Can you work these out from the model? Positions are in its coordinate system, mm. Face numbers are marked on the shaded views. Round coordinates to 2 decimals unless told otherwise and drop trailing zeros. Write each loop counter-clockwise with the first axis right and the second up, starting at its lowest first coordinate (ties: lowest second). Pieces come first, ordered by that corner, then holes.
Q1. I'm going to push flat-ended pins straight in: pin 1 Ø1.5 at (x, z) = (6.5, -12) entering from +Y; pin 2 Ø5 at (x, z) = (-2, -4) entering from +Y; pin 3 Ø5 at (y, z) = (7.5, -4.5) entering from -X. Where does each tip first touch, or does it pass through?
Q2. If we section it at A-A (x = 0): Please give me the cut outline in (y, z).
Q3. If we section it at D-D (y = -10): Please give me the cut outline in (x, z), plus the area to 3 significant figures.
Q4. We'd pull the mould along X, two halves only. Please class the marked faces 1, 2 and 3: +X half, -X half, draft (parallel to the pull), parting line (faces both ways), or undercut.
Q5. Please list where these lines run through material, in increasing order: line 1 along Y through (x, z) = (0, -5); line 2 along Z through (x, y) = (0, 21.5); line 3 along X through (y, z) = (0.5, -7).
Q6. If we section it at C-C (z = -1): Please give me the cut outline in (x, y), plus the area to 3 significant figures.
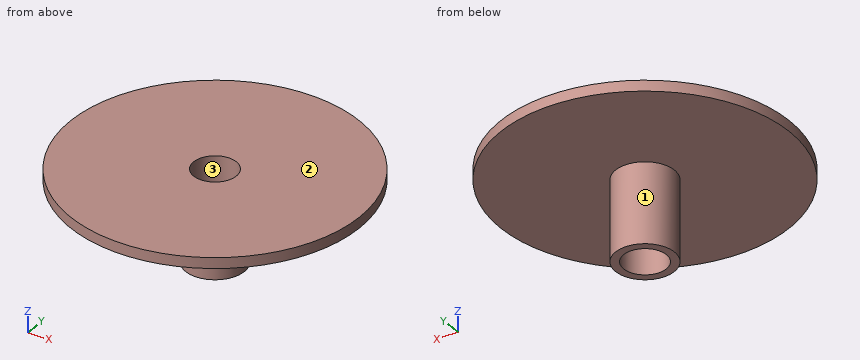
from build123d import *

# Parameters (mm, degrees)
SKETCH_1_R          = 27
EXTRUDE_1_DEPTH     = 2
SKETCH_2_R          = 5.5
EXTRUDE_2_DEPTH     = 15
SKETCH_3_R          = 4
CUT_EXTRUDE_1_DEPTH = 150


with BuildPart() as part:
    # 草图1 → 凸台-拉伸1 (new body)
    with BuildSketch(Plane.XY):
        Circle(SKETCH_1_R)
    extrude(amount=EXTRUDE_1_DEPTH)

    # 草图2 → 凸台-拉伸2 (add)
    with BuildSketch(Plane.XY):
        Circle(SKETCH_2_R)
    extrude(amount=-EXTRUDE_2_DEPTH)

    # 草图3 → 切除-拉伸1 (cut)
    with BuildSketch(Plane(origin=(0, 0, -15), x_dir=(-1, 0, 0), z_dir=(0, 0, -1))):
        Circle(SKETCH_3_R)
    extrude(amount=-CUT_EXTRUDE_1_DEPTH, mode=Mode.SUBTRACT)


solid = part.part
A:
1. pin 1: passes through
1. pin 2: stops at y = 5.5
1. pin 3: stops at x = -2.29
2. outline: (-27, 0) - (-5.5, 0) - (-5.5, -15) - (-4, -15) - (-4, 2) - (-27, 2) - close; (4, -15) - (5.5, -15) - (5.5, 0) - (27, 0) - (27, 2) - (4, 2) - close
3. outline: (-25.08, 0) - (25.08, 0) - (25.08, 2) - (-25.08, 2) - close
3. area: 100 mm2
4. face 1: parting line
4. face 2: draft
4. face 3: undercut
5. line 1: y = -5.5 to -4, 4 to 5.5
5. line 2: z = 0 to 2
5. line 3: x = -5.48 to -3.97, 3.97 to 5.48
6. outline: circle Ø11 at (0, 0); hole circle Ø8 at (0, 0)
6. area: 44.8 mm2
